Geometry: final body of the model. Coordinates: model frame, mm. A direction names the side the tool comes from. Coordinates: 2 decimals unless noted, no trailing zeros. Order: outer loops, then holes, each group sorted by start corner. A loop starts at its lowest first (then second) coordinate and runs counter-clockwise, first axis right, second up. Notation, with made-up numbers: M 8,81.5 L 49,81.5 A22 cw 49,109.5 Z; hole C 26.25,-24.5 d9. An arc over 180 degrees is marked long. Write item = value, one per line.
from build123d import *

# Parameters (mm, degrees)
BOSS_EXTRUDE1_DEPTH  = 3.175
SKETCH2_W            = 6.35
SKETCH2_H            = 12.7
CUT_EXTRUDE1_DEPTH   = 2.54
LPATTERN1_COUNT      = 5
LPATTERN1_PITCH      = 9.652
LPATTERN1_COUNT_DIR2 = 7
LPATTERN1_PITCH_DIR2 = 15.24


with BuildPart() as part:
    # Sketch1 → Boss-Extrude1 (new body)
    with BuildSketch(Plane.XY):
        Polygon((0, -152.4), (12.7, -152.4), (38.1, -152.4), (50.8, -152.4), (50.8, -139.7), (47.625, -139.7), (47.625, -133.35), (50.8, -133.35), (50.8, -19.05), (47.625, -19.05), (47.625, -12.7), (50.8, -12.7), (50.8, 0), (38.1, 0), (38.1, -3.175), (31.75, -3.175), (31.75, 0), (19.05, 0), (19.05, -3.175), (12.7, -3.175), (12.7, 0), (0, 0), (0, -12.7), (3.175, -12.7), (3.175, -19.05), (0, -19.05), (0, -133.35), (3.175, -133.35), (3.175, -139.7), (0, -139.7), align=None)
    extrude(amount=BOSS_EXTRUDE1_DEPTH)

    # Sketch2 → Cut-Extrude1 (cut)
    with BuildSketch(Plane.XY.offset(3.175)):
        with Locations((6.477, -31.75)):
            Rectangle(SKETCH2_W, SKETCH2_H)
    cut_extrude1 = extrude(amount=-CUT_EXTRUDE1_DEPTH, mode=Mode.SUBTRACT)

    # LPattern1: Cut-Extrude1 5 × 7
    with Locations(*[(i * LPATTERN1_PITCH, -j * LPATTERN1_PITCH_DIR2, 0) for i in range(LPATTERN1_COUNT) for j in range(LPATTERN1_COUNT_DIR2) if (i, j) != (0, 0)]):
        add(cut_extrude1, mode=Mode.SUBTRACT)


solid = part.part
1) Mould query, pull axis Y, two halves, no side actions, for faces 3 (the face through (0, -75, 2)), 4 (the face through (48.26, -32, 2)), 5 (the face through (48.26, -78, 2)). Classes: pulls with the +Y half, pulls with the -Y half, needs draft (parallel to the pull), parting line crosses it, or undercut.
Numbers:
face_3 = needs draft
face_4 = undercut
face_5 = undercut
2) Pin query (flat end, axial travel): pin 1 (1.9 mm diameter, centred on x = 46.5, y = -92, fed in from +Z) (3 decimals). Return the tip coordinate at first contact, or that it passes through.
Numbers:
pin_1 = 0.635
3) Set-up query: faces 1 (the face through (26, -116.84, 2)), 2 (the face through (2, -133.35, 2)). Return all of +Z, -Z, +X, -X, +Y, -Y with unobstructed straight access to the full face (end or side cutting, diameter ignored); none if empty.
Numbers:
face_1 = +Z
face_2 = +Z, -Z, -X
4) Section C-C, the plane z = 1.75. Give the number of separate pieces and of enclosed holes in the cut face, and give its area (3 significant figures).
Numbers:
separate_pieces = 1
enclosed_holes = 35
area = 4,800 mm²
5) Section D-D, the plane y = -17.5. Return loops of the section in (x, z) (3 decimals), and give its area (3 significant figures).
Numbers:
outline = M 3.175,0 L 47.625,0 L 47.625,3.175 L 3.175,3.175 Z
area = 141 mm²
6) Line query: L1, parallel to X at y = -47.5, z = 1.7; L2, parallel to Z at x = 38, y = -60 (3 decimals); L3, parallel to X at y = -17, z = 1.8 (3 decimals). Output: solid intervals per line, ascending.
Numbers:
L1 = 0 to 3.3, 9.65 to 12.95, 19.3 to 22.61, 28.96 to 32.26, 38.61 to 41.91, 48.26 to 50.8
L2 = 0 to 0.635
L3 = 3.175 to 47.625
7) Section A-A, the plane y = -57.5. Return loops of the section in (x, z) (3 decimals).
Numbers:
outline = M 0,0 L 50.8,0 L 50.8,3.175 L 48.26,3.175 L 48.26,0.635 L 41.91,0.635 L 41.91,3.175 L 38.608,3.175 L 38.608,0.635 L 32.258,0.635 L 32.258,3.175 L 28.956,3.175 L 28.956,0.635 L 22.606,0.635 L 22.606,3.175 L 19.304,3.175 L 19.304,0.635 L 12.954,0.635 L 12.954,3.175 L 9.652,3.175 L 9.652,0.635 L 3.302,0.635 L 3.302,3.175 L 0,3.175 Z
